Print and shaded views of the part. All mm, measured from the part's lowest x, y and z. A direction names the side the tool comes from. Coordinates: 2 decimals unless noted, no trailing zeros. Order: outer loops, then holes, each group sorted by start corner. A loop starts at its lowest first (then second) coordinate and runs counter-clockwise, first axis right, second up.
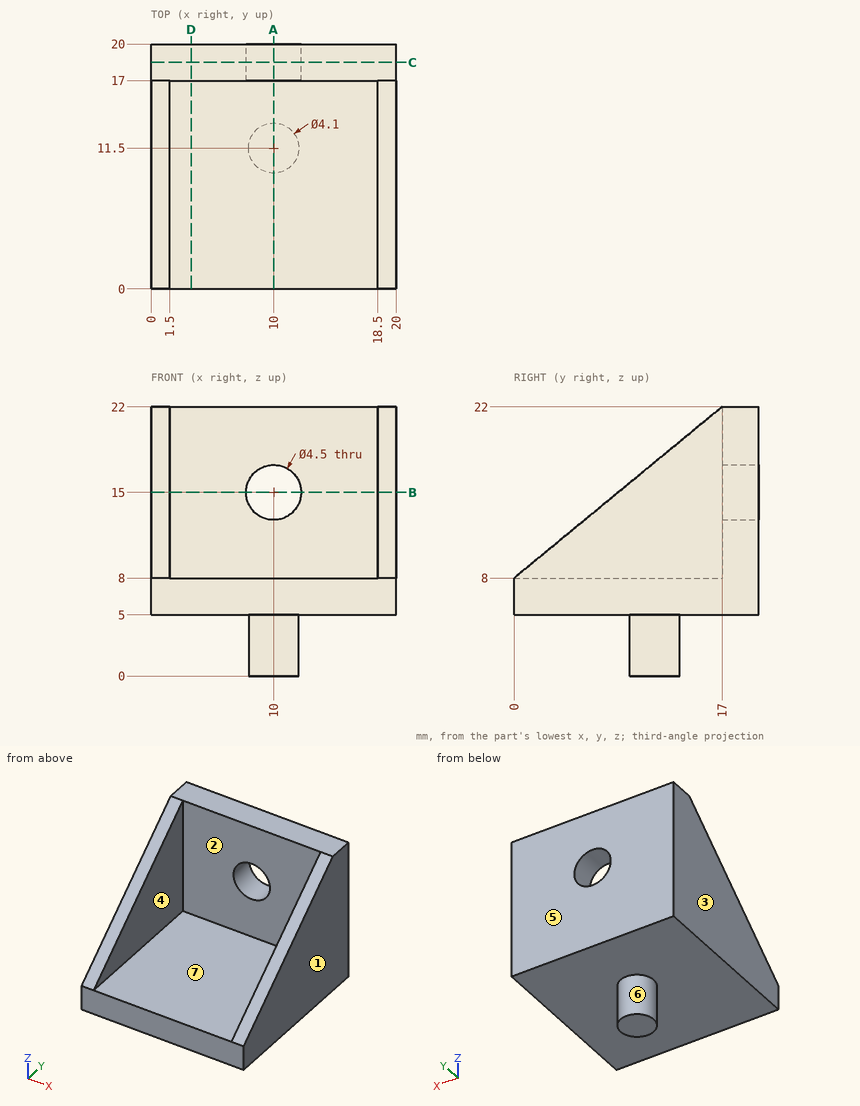
Q1. Cut at C-C, the plane y = 18.5. List the corners of the cut face in (x, z).
Established:
outline: (0, 5) - (20, 5) - (20, 22) - (0, 22) - close; hole circle Ø4.5 at (10, 15)
Q2. Drop flat-ended pins along their axis: P1, Ø6, axis at x = 12, y = 3.5, coming from the +Z side; P2, Ø4, axis at x = 17, y = 3.5, coming from the +Z side. Give the stop position or say it passes through.
Established:
P1: stops at z = 8
P2: stops at z = 11.97
Q3. Cut at D-D, the plane x = 3.25. List the corners of the cut face in (y, z).
Established:
outline: (0, 5) - (20, 5) - (20, 22) - (17, 22) - (17, 8) - (0, 8) - close
Q4. Probe line 1 (Z direction, x = 10, y = 18.8); line 2 (X direction, y = 13, z = 11.5); line 3 (Z direction, x = 6.75, y = 4). List the from-to ranges inside material, lowest first.
Established:
line 1: z = 5 to 12.75, 17.25 to 22
line 2: x = 0 to 1.5, 18.5 to 20
line 3: z = 5 to 8
Q5. Cut at A-A, the plane x = 10. List the corners of the cut face in (y, z).
Established:
outline: (0, 5) - (9.45, 5) - (9.45, 0) - (13.55, 0) - (13.55, 5) - (20, 5) - (20, 12.75) - (17, 12.75) - (17, 8) - (0, 8) - close; (17, 17.25) - (20, 17.25) - (20, 22) - (17, 22) - close
Q6. Which spindle directions (+Z, -Z, +X, -X, +Y, -Y) get a long thin tool onto all of the face, cutting with end or side? Do the marked faces 5, 6 and 7. Say none if no direction does.
Established:
face 5: +Z, -Z, +X, -X, +Y
face 6: -Z
face 7: +Z, -Y
Q7. Mould opens along X. For the marked faces 1, 2, 3 and 4 say: pulls with the +X half, pulls with the -X half, needs draft (parallel to the pull), parting line crosses it, or undercut.
Established:
face 1: pulls with the +X half
face 2: undercut
face 3: pulls with the -X half
face 4: undercut
Q8. Cut at B-B, the plane z = 15. List the corners of the cut face in (x, y).
Established:
outline: (0, 8.5) - (1.5, 8.5) - (1.5, 17) - (7.75, 17) - (7.75, 20) - (0, 20) - close; (12.25, 17) - (18.5, 17) - (18.5, 8.5) - (20, 8.5) - (20, 20) - (12.25, 20) - close
